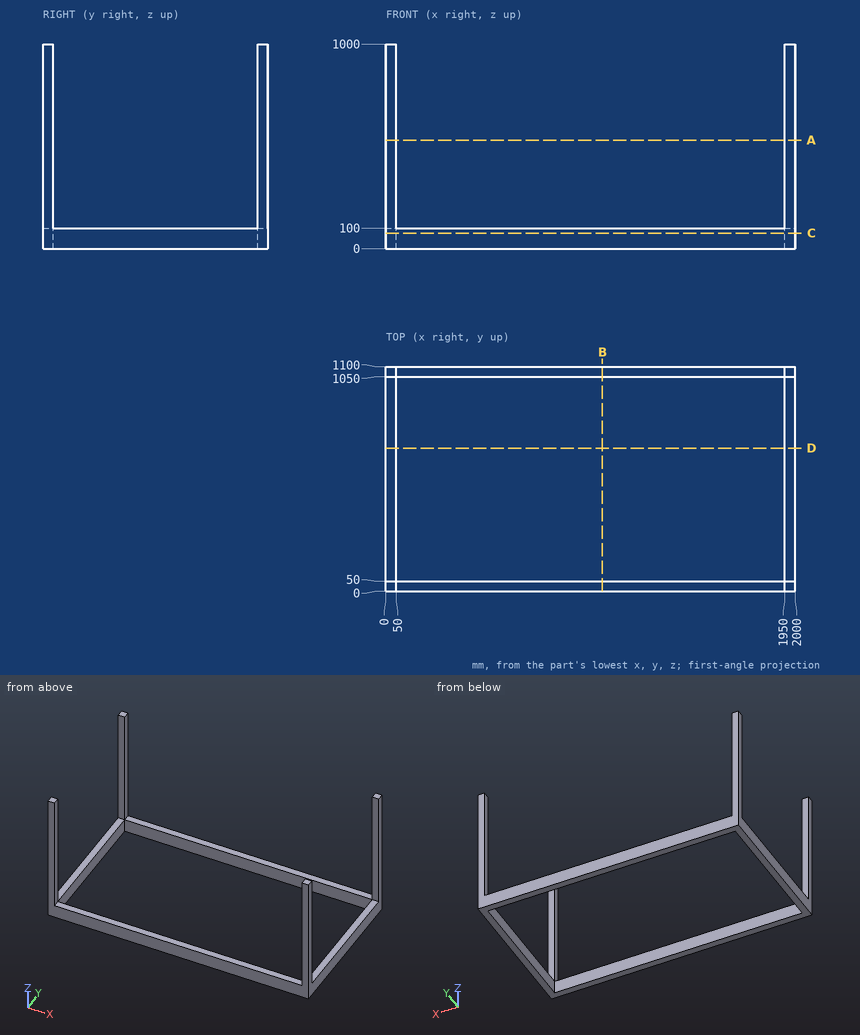
Design review of the part shown in the three views and the two pictorial views. Dimensions are in mm from the part's minimum x, y and z. Give positions to 0.01 mm unless a question says otherwise; leave off trailing zeros. Loops run counter-clockwise (first coordinate to the right, second up) from the corner with the lowest first, then second, coordinate; pieces in that order, holes last. Notation, with made-up numbers: (-33, -1.5) -> (-23, -1.5) arc R27 cw to (-23, 26.5) -> close; hole circle Ø9 at (-34, 8). An arc over 180 degrees is marked (long way). Write each question's results on one line, items separated by ' | '.
Q1. Take a section at A-A, the plane z = 529.5. Write out the cut boundary in (x, y), plus the area to 3 significant figures.
Reply:
outline: (0, 0) -> (50, 0) -> (50, 50) -> (0, 50) -> close; (0, 1050) -> (50, 1050) -> (50, 1100) -> (0, 1100) -> close; (1950, 0) -> (2000, 0) -> (2000, 50) -> (1950, 50) -> close; (1950, 1050) -> (2000, 1050) -> (2000, 1100) -> (1950, 1100) -> close | area: 10,000 mm²
Q2. Take a section at B-B, the plane x = 1058.5. Write out the cut boundary in (y, z), plus the area to 3 significant figures.
Reply:
outline: (0, 0) -> (50, 0) -> (50, 100) -> (0, 100) -> close; (1050, 0) -> (1100, 0) -> (1100, 100) -> (1050, 100) -> close | area: 10,000 mm²
Q3. For pin 1 Ø25 at (x, y) = (1971, 464.5) entering from +Z, flat-tipped, find the tip position at first contact; note if it passes through.
Reply:
pin 1: stops at z = 100
Q4. Take a section at D-D, the plane y = 700.5. Write out the cut boundary in (x, z).
Reply:
outline: (0, 0) -> (50, 0) -> (50, 100) -> (0, 100) -> close; (1950, 0) -> (2000, 0) -> (2000, 100) -> (1950, 100) -> close
Q5. Take a section at C-C, the plane z = 75.5. Write out the cut boundary in (x, y).
Reply:
outline: (0, 0) -> (2000, 0) -> (2000, 1100) -> (0, 1100) -> close; hole (50, 50) -> (1950, 50) -> (1950, 1050) -> (50, 1050) -> close
Q6. Wall thickness on L1, parallel to X at y = 813.5, z = 41.5; L2, parallel to Y at x = 1827, z = 80.5: over which ranges is each line inside the solid? List them lowest first.
Reply:
L1: x = 0 to 50, 1950 to 2000 | L2: y = 0 to 50, 1050 to 1100
